Autodesk Inventor part; units mm, degrees
ref_plane "YZ Plane" through (0, 0, 0) normal (1, 0, 0) x (0, 1, 0)
ref_plane "XZ Plane" through (0, 0, 0) normal (0, 1, 0) x (-1, 0, 0)
ref_plane "XY Plane" through (0, 0, 0) normal (0, 0, 1) x (1, 0, 0)
sketch "S-Base" plane through (0, 0, 0) normal (0, 1, 0) x (-1, 0, 0)
  line L0 (0, 0) -> (11, 0)
  line L1 (11, 0) -> (11, -34.4)
  line L2 (11, -34.4) -> (0, -34.4)
  line L3 (0, -34.4) -> (0, 0)
  circle A0 centre (4, -17.2) radius 3.5
  line L4 (0, -14.1) -> (7.5, -14.1)
  line L5 (7.5, -14.1) -> (7.5, -20.3)
  line L6 (7.5, -20.3) -> (0, -20.3)
  line L7 (0, -20.3) -> (0, -14.1) construction
  line L8 (7.5, -17.2) -> (0, -17.2) construction
  circle A1 centre (4, -17.2) radius 3.75
  point P0 (6.1101, -20.3)
  point P1 (0, -20.3)
  point P2 (6.1101, -14.1)
  dimension "d1" = 7
  dimension "d0" = 34.4
  dimension "d2" = 17.2
  dimension "d3" = 6.2
  dimension "d4" = 11
  dimension "d5" = 7.5
  dimension "d6" = 0.25
extrude "Ex-Base" add sketch "S-Base" along normal blind 2.5 contours L0 L1 L2 L3 L6 A1 L5 L4 | A1 L4 A0 | L6 A0 A1 | A0 L4 | L4 L5 A1 | L6 A0 | A1 L5 L6
chamfer "Fase1" distance 0.5 angle 45 12 edges at (-11, 1.25, 0) (0, 1.25, 0) (0, 1.25, -34.4) (-11, 1.25, -34.4) (0, 1.25, -20.3) (0, 1.25, -14.1) (-11, 2.5, -17.2) (-11, 0, -17.2) (0, 2.5, -7.05) (0, 0, -7.05) (0, 2.5, -27.35) (0, 0, -27.35)
equation "\"d2\" = 0.5 * d0"
properties part number "ProbeHead_Kabelfixieung_V2"
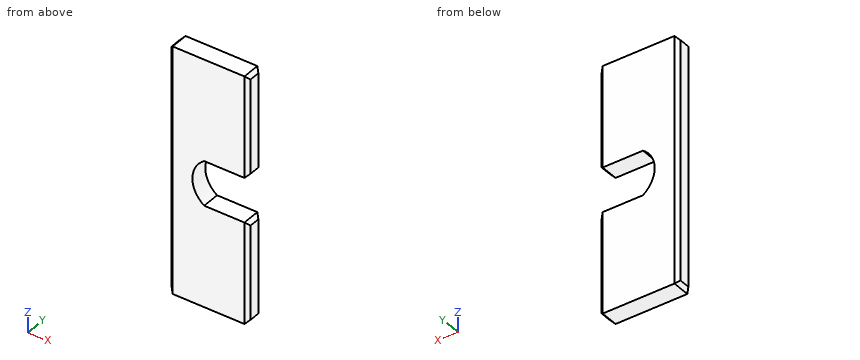
Model file for the job. Use its own axes, mm. Give positions to 0.01 mm unless a question says otherwise; leave off trailing zeros. Order: outer loops, then holes, each group sorted by start corner. A loop starts at its lowest first (then second) coordinate and runs counter-clockwise, first axis right, second up. Notation, with made-up numbers: M 25,19 L 69,19 A25 ccw 69,55 Z; hole C 58.5,10 d11. An arc over 180 degrees is marked long. Put each result on its own line as item: value. Start each with the question number.
(1) Band-saw the part on A-A on x = -2.75. Give the cut face in (y, z).
(2) Band-saw the part on D-D on x = -6.5. Give the cut face in (y, z), then the cut area to 3 significant figures.
(3) Drill centre lines: L1, parallel to Z at x = -4.75, y = 1.4; L2, parallel to Z at x = -7, y = 0.7; L3, parallel to X at y = 1.75, z = -17. Where is each one in solid material? Low to high. Write a range as [from, to].
(4) Band-saw the part on C-C on y = 1.7. Give the cut face in (x, z).
(5) Band-saw the part on B-B on z = -25. Give the cut face in (x, y), then the cut area to 3 significant figures.
Results below:
1. outline: M 0,-34.4 L 2.5,-34.4 L 2.5,-20.3 L 0,-20.3 Z; M 0,-14.1 L 2.5,-14.1 L 2.5,0 L 0,0 Z
2. outline: M 0,-34.4 L 2.5,-34.4 L 2.5,-20 L 0,-20 Z; M 0,-14.4 L 2.5,-14.4 L 2.5,0 L 0,0 Z
2. area: 72.0 mm2
3. L1: z = [-34.4, -20.3], [-14.1, 0]
3. L2: z = [-34.4, -19.45], [-14.95, 0]
3. L3: x = [-11, -7.74]
4. outline: M -11,-33.9 L -10.5,-34.4 L -0.5,-34.4 L 0,-33.9 L 0,-20.8 L -0.5,-20.3 L -6.11,-20.3 A3.75 cw -6.11,-14.1 L -0.5,-14.1 L 0,-13.6 L 0,-0.5 L -0.5,0 L -10.5,0 L -11,-0.5 Z
5. outline: M -11,0.5 L -10.5,0 L -0.5,0 L 0,0.5 L 0,2 L -0.5,2.5 L -10.5,2.5 L -11,2 Z
5. area: 27.0 mm2
